The listing builds one solid part. Answer for the finished solid, in the listing's coordinates (mm). A direction names the side the tool comes from. Round coordinates to 2 decimals unless told otherwise and drop trailing zeros. Order: outer loops, then holes, each group sorted by start corner. A loop starts at its lowest first (then second) coordinate and runs counter-clockwise, first axis right, second up. Notation, with made-up numbers: (-16, 42.5) -> (31, 42.5) arc R35 ccw to (31, 76.5) -> close; hole circle Ø2 at (41, 37). An arc over 180 degrees is marked (long way). Return JSON: item names as keys, results as strings. Group by question number.
(1) Consider line 1 (X direction, y = 5, z = 6.5); line 2 (Y direction, x = 8.25, z = 8); line 3 (Z direction, x = 8, y = 7.75). Determine where each line is inside the solid, lowest interval first. Write a range as [from, to].
(2) Which of the six approach directions +Z, -Z, +X, -X, +Y, -Y give full straight-line access (tool end or side, diameter ignored) to faces 1 (the face through (6, 1, 6)), 2 (the face through (9, 1.5, 5)), 3 (the face through (5, 5, 0))?
(3) The part is cut by section C-C (z = 4.25). Count the separate pieces of the cut face and the enclosed holes in it, plus the area to 3 significant figures.
(4) The part is cut by section B-B (y = 4.5). Determine the outline of the cut face in (x, z).
(5) The part is cut by section A-A (x = 3). Determine the outline of the cut face in (y, z).
(6) Determine the mould class of faces 4 (the face through (5, 0, 4)), 5 (the face through (0, 5, 4)), 6 (the face through (4, 9, 6)) for opening direction X: +X half, -X half, draft (parallel to the pull), parting line (faces both ways), or undercut.
from build123d import *

# Parameters (mm, degrees)
F0_W     = 10
F0_H     = 10
F1_DEPTH = 1.7
F2_SIZE  = 0.25
F3_W     = 2
F3_H     = 1.5
F4_DEPTH = 8.3
F5_R     = 0.74999


# Not quite as in the source:
# - a fillet or chamfer is up to 0.001 mm smaller than in the source, because OpenCascade refuses the exact size


with BuildPart() as f1:
    # F0 (on Top) → F1 (new body)
    with BuildSketch(Plane.XY):
        with Locations((5, 5)):
            Rectangle(F0_W, F0_H)
    extrude(amount=F1_DEPTH)

    # F2
    f2_edges = [f1.edges().sort_by_distance(p)[0] for p in [
        (5, 0, 0),
        (0, 5, 0),
        (10, 5, 0),
        (5, 10, 0),
    ]]
    chamfer(f2_edges, length=F2_SIZE)

    # F3 (on face) → F4 (join)
    with BuildSketch(Plane.XY.offset(1.7)):
        with Locations((1, 9.25)):
            Rectangle(F3_W, F3_H)
        with Locations((9, 9.25)):
            Rectangle(F3_W, F3_H)
        with Locations((1, 0.75)):
            Rectangle(F3_W, F3_H)
        with Locations((9, 0.75)):
            Rectangle(F3_W, F3_H)
        with Locations((1, 5)):
            Rectangle(F3_W, F3_H)
        with Locations((5, 9.25)):
            Rectangle(F3_W, F3_H)
        with Locations((9, 5)):
            Rectangle(F3_W, F3_H)
        with Locations((5, 5)):
            Rectangle(F3_W, F3_H)
        with Locations((5, 0.75)):
            Rectangle(F3_W, F3_H)
    extrude(amount=F4_DEPTH)

    # F5 (radius 0.75 in the source; OpenCascade refuses exactly that, so slightly less here)
    f5_edges = [f1.edges().sort_by_distance(p)[0] for p in [
        (1, 0, 10),
        (1, 1.5, 10),
        (5, 0, 10),
        (9, 0, 10),
        (9, 1.5, 10),
        (9, 4.25, 10),
        (9, 5.75, 10),
        (5, 4.25, 10),
        (5, 5.75, 10),
        (1, 4.25, 10),
        (1, 5.75, 10),
        (1, 8.5, 10),
        (1, 10, 10),
        (5, 8.5, 10),
        (5, 10, 10),
        (9, 8.5, 10),
        (9, 10, 10),
    ]]
    fillet(f5_edges, radius=F5_R)


solid = f1.part
Answer below:
{
 "1": {"line 1": "x = [0, 2], [4, 6], [8, 10]", "line 2": "y = [0, 1.5], [4.25, 5.75], [8.5, 10]", "line 3": "z = [0, 1.7]"},
 "2": {"face 1": "+Z, +Y, -Y", "face 2": "+Z, +X, -X", "face 3": "-Z, +X, -X, +Y, -Y"},
 "3": {"separate pieces": "9", "enclosed holes": "0", "area": "27.0 mm²"},
 "4": {"outline": "(0, 0.25) -> (0.25, 0) -> (9.75, 0) -> (10, 0.25) -> (10, 9.81) -> (8, 9.81) -> (8, 1.7) -> (6, 1.7) -> (6, 9.81) -> (4, 9.81) -> (4, 1.7) -> (2, 1.7) -> (2, 9.81) -> (0, 9.81) -> close"},
 "5": {"outline": "(0, 0.25) -> (0.25, 0) -> (9.75, 0) -> (10, 0.25) -> (10, 1.7) -> (0, 1.7) -> close"},
 "6": {"face 4": "draft", "face 5": "-X half", "face 6": "undercut"}
}
